Input: part model. Units: mm. Frame: model coordinates. A direction names the side the tool comes from. Give positions to 0.01 mm unless a question says otherwise; leave off trailing zeros. Order: outer loops, then holes, each group sorted by start corner. A loop starts at its lowest first (then second) coordinate and runs counter-clockwise, first axis right, second up. Notation, with made-up numbers: (-30.75, -17) - (18.25, -17) arc R23 ccw to (18.25, -1) - close; hole circle Ø9 at (-11, 15.25). An arc over 180 degrees is marked (long way). Answer in a Markdown table with one row per item. Add a question column.
from build123d import *

# Parameters (mm, degrees)
ESQUISSE3_W             = 50
ESQUISSE3_H             = 40
BOSS_EXTRU_1_DEPTH      = 22.5
ESQUISSE7_W             = 30
ESQUISSE7_H             = 20
ENL_V_MAT_EXTRU_1_DEPTH = 78.551730665
ESQUISSE8_W             = 5
ESQUISSE8_H             = 40
ENL_V_MAT_EXTRU_2_DEPTH = 20
ESQUISSE9_W             = 15
ESQUISSE9_H             = 10
ENL_V_MAT_EXTRU_3_DEPTH = 10
CHANFREIN2_SIZE         = 10
CHANFREIN3_SIZE         = 10
ENL_V_MAT_EXTRU_4_DEPTH = 109.911404208
ESQUISSE11_W            = 20
ESQUISSE11_H            = 15
ENL_V_MAT_EXTRU_5_DEPTH = 25
ESQUISSE12_W            = 10
ESQUISSE12_H            = 15
ENL_V_MAT_EXTRU_6_DEPTH = 25
ESQUISSE14_R            = 3
ENL_V_MAT_EXTRU_7_DEPTH = 95.127164185
ESQUISSE15_R            = 5
ENL_V_MAT_EXTRU_8_DEPTH = 109.911404208


with BuildPart() as part:
    # Esquisse3 → Boss.-Extru.1 (new, symmetric)
    with BuildSketch(Plane.XY):
        with Locations((-64.183367493, -34.845427604)):
            Rectangle(ESQUISSE3_W, ESQUISSE3_H)
    extrude(amount=BOSS_EXTRU_1_DEPTH, both=True)

    # Esquisse7 → Enlèv. mat.-Extru.1 (cut, through all)
    with BuildSketch(Plane(origin=(-39.183367493, 0, 0), x_dir=(0, 0, -1), z_dir=(1, 0, 0))):
        with Locations((7.5, -24.845427604)):
            Rectangle(ESQUISSE7_W, ESQUISSE7_H)
    extrude(amount=-ENL_V_MAT_EXTRU_1_DEPTH, mode=Mode.SUBTRACT)

    # Esquisse8 → Enlèv. mat.-Extru.2 (cut)
    with BuildSketch(Plane(origin=(-39.183367493, 0, 0), x_dir=(0, 0, -1), z_dir=(1, 0, 0))):
        with Locations((-20, -34.845427604)):
            Rectangle(ESQUISSE8_W, ESQUISSE8_H)
    extrude(amount=-ENL_V_MAT_EXTRU_2_DEPTH, mode=Mode.SUBTRACT)

    # Esquisse9 → Enlèv. mat.-Extru.3 (cut)
    with BuildSketch(Plane.ZY.offset(89.183367493)):
        with Locations((-15, -39.845427604)):
            Rectangle(ESQUISSE9_W, ESQUISSE9_H)
    extrude(amount=-ENL_V_MAT_EXTRU_3_DEPTH, mode=Mode.SUBTRACT)

    # Chanfrein2
    chanfrein2_edges = [part.edges().sort_by_distance(p)[0] for p in [
        (-39.183367493, -14.845427604, 12.5),
    ]]
    chamfer(chanfrein2_edges, length=CHANFREIN2_SIZE)

    # Chanfrein3
    chanfrein3_edges = [part.edges().sort_by_distance(p)[0] for p in [
        (-39.183367493, -44.845427604, -22.5),
    ]]
    chamfer(chanfrein3_edges, length=CHANFREIN3_SIZE)

    # Esquisse10 → Enlèv. mat.-Extru.4 (cut, through all)
    with BuildSketch(Plane(origin=(0, 0, 7.5), x_dir=(-1, 0, 0), z_dir=(0, 0, -1))):
        Polygon((74.183367493, -14.845427604), (79.183367493, -14.845427604), (79.183367493, -21.845427604), (84.183367493, -21.845427604), (84.183367493, -26.845427604), (69.183367493, -26.845427604), (69.183367493, -21.845427604), (74.183367493, -21.845427604), align=None)
    extrude(amount=-ENL_V_MAT_EXTRU_4_DEPTH, mode=Mode.SUBTRACT)

    # Esquisse11 → Enlèv. mat.-Extru.5 (cut)
    with BuildSketch(Plane(origin=(-39.183367493, 0, 0), x_dir=(0, 0, -1), z_dir=(1, 0, 0))):
        with Locations((-2.5, -47.345427604)):
            Rectangle(ESQUISSE11_W, ESQUISSE11_H)
    extrude(amount=-ENL_V_MAT_EXTRU_5_DEPTH, mode=Mode.SUBTRACT)

    # Esquisse12 → Enlèv. mat.-Extru.6 (cut)
    with BuildSketch(Plane(origin=(0, 0, -22.5), x_dir=(-1, 0, 0), z_dir=(0, 0, -1))):
        with Locations((59.183367493, -47.345427604)):
            Rectangle(ESQUISSE12_W, ESQUISSE12_H)
    extrude(amount=-ENL_V_MAT_EXTRU_6_DEPTH, mode=Mode.SUBTRACT)

    # Esquisse14 → Enlèv. mat.-Extru.7 (cut, through all)
    with BuildSketch(Plane(origin=(0, -34.845427604, 0), x_dir=(1, 0, 0), z_dir=(0, 1, 0))):
        with Locations(Location((-74.183367493, 3.5, 0), (0, 0, 270))):
            Circle(ESQUISSE14_R)
    extrude(amount=-ENL_V_MAT_EXTRU_7_DEPTH, mode=Mode.SUBTRACT)

    # Esquisse15 → Enlèv. mat.-Extru.8 (cut, through all)
    with BuildSketch(Plane(origin=(0, 0, 7.5), x_dir=(-1, 0, 0), z_dir=(0, 0, -1))):
        with Locations((57.183367493, -24.845427604)):
            Circle(ESQUISSE15_R)
    extrude(amount=-ENL_V_MAT_EXTRU_8_DEPTH, mode=Mode.SUBTRACT)


solid = part.part
Q1. Contact query for flat-ended pins moving along their axis: P1, Ø15, axis at x = -58, z = -1.5, coming from the +Y side; P2, Ø5, axis at y = -38, z = -18, coming from the -X side; P3, Ø8, axis at y = -28.5, z = -9, coming from the -X side; P4, Ø5.5, axis at y = -18, z = 18.5, coming from the +X side. Output: stop coordinate, or through.
Q2. Section D-D, the plane z = 16. Return loops of the section in (x, y), then the cut area to 3 significant figures.
Q3. Section A-A, the plane z = -3.5. Return loops of the section in (x, y).
Q4. Pull-direction query (X, two-part tool) for faces 4 (the flat face through (-59.183, -42, 20)), 5 (the flat face through (-64.183, -47, -5)), 6 (the flat face through (-48, -54.845, -13)), 7 (the flat face through (-84.183, -24, 15)); classes: +X half, -X half, draft (parallel to the pull), parting line (faces both ways), or undercut.
Q5. Line query: probe 1 along Y at (x, z) = (-79.5, 10.5); probe 2 along X at (y, z) = (-45, -11.5); probe 3 along X at (y, z) = (-41.75, -3.5). Output: solid intervals per line, ascending.
Q6. Access query for faces 1 (the flat face through (-82, -21.845, 15)), 2 (the flat face through (-47, -47, -7.5)), 3 (the flat face through (-64, -34.845, -7)). Directions: +Z, -Z, +X, -X, +Y, -Y. A direction counts if a zero-diameter tool reaches every point of the face in a straight line with its end or side. Return the directions, or none.
Q7. Section B-B, the plane y = -43. Return loops of the section in (x, z).
Q8. Section C-C, the plane x = -70.5. Return loops of the section in (y, z), then the cut area to 4 significant figures.
Computed:
| question | item | result |
|---|---|---|
| 1 | P1 | stops at y = -34.85 |
| 1 | P2 | stops at x = -79.18 |
| 1 | P3 | passes through |
| 1 | P4 | stops at x = -43.47 |
| 2 | outline | (-89.18, -54.85) - (-39.18, -54.85) - (-39.18, -24.85) - (-49.18, -14.85) - (-74.18, -14.85) - (-74.18, -21.85) - (-69.18, -21.85) - (-69.18, -26.85) - (-84.18, -26.85) - (-84.18, -21.85) - (-79.18, -21.85) - (-79.18, -14.85) - (-89.18, -14.85) - close; hole circle Ø10 at (-57.18, -24.85) |
| 2 | area | 1,760 mm^2 |
| 3 | outline | (-89.18, -54.85) - (-77.18, -54.85) - (-77.18, -34.85) - (-89.18, -34.85) - close; (-71.18, -54.85) - (-64.18, -54.85) - (-64.18, -39.85) - (-39.18, -39.85) - (-39.18, -34.85) - (-71.18, -34.85) - close |
| 4 | face 4 | +X half |
| 4 | face 5 | undercut |
| 4 | face 6 | draft |
| 4 | face 7 | undercut |
| 5 | probe 1 | y = -54.85 to -26.85, -21.85 to -14.85 |
| 5 | probe 2 | x = -89.18 to -64.18, -54.18 to -39.18 |
| 5 | probe 3 | x = -89.18 to -77.18, -71.18 to -64.18 |
| 6 | face 1 | +Z, -Z |
| 6 | face 2 | +X, -Y |
| 6 | face 3 | -Z, +X, -X, +Y |
| 7 | outline | (-89.18, -7.5) - (-79.18, -7.5) - (-79.18, -22.5) - (-64.18, -22.5) - (-64.18, 12.5) - (-39.18, 12.5) - (-39.18, 17.5) - (-59.18, 17.5) - (-59.18, 22.5) - (-89.18, 22.5) - close; (-54.18, -22.5) - (-49.18, -22.5) - (-39.18, -12.5) - (-39.18, -7.5) - (-54.18, -7.5) - close; hole circle Ø6 at (-74.18, -3.5) |
| 8 | outline | (-54.85, -22.5) - (-34.85, -22.5) - (-34.85, 7.5) - (-26.85, 7.5) - (-26.85, 22.5) - (-54.85, 22.5) - close; (-21.85, 7.5) - (-14.85, 7.5) - (-14.85, 22.5) - (-21.85, 22.5) - close |
| 8 | area | 1,125 mm^2 |
